Build history of the part. All positions in model axes, mm. Face numbers are marked on the shaded views. Round coordinates to 2 decimals unless told otherwise and drop trailing zeros. Loops run counter-clockwise (first coordinate to the right, second up) from the corner with the lowest first, then second, coordinate; pieces in that order, holes last. Notation, with made-up numbers: (50.25, -3) - (74.25, -3) arc R25 cw to (74.25, 21) - close; hole circle Ø6 at (-17, -36.75). An arc over 180 degrees is marked (long way). Use a Markdown table: item, result.
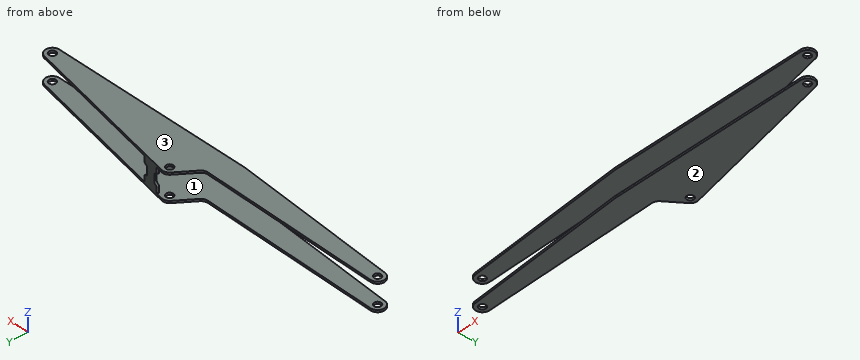
from build123d import *

# Parameters (mm, degrees)
PROFILE_EXTRUDE_DEPTH        = 40
LIGHTNING_BOLT_FILLET_R      = 10
SHELL_CUT_REACH              = 291.378
SHELL_SKETCH_W               = 549.904110801
SHELL_SKETCH_H               = 34
HOLES_START                  = -40
HOLES_SKETCH_R               = 5
HOLES_CUT_DEPTH              = 40
BOWTIE_SUPPORT_EXTRUDE_DEPTH = 3
BOWTIE_SUPPORT_FILLET_R      = 2.5


# Some blends are built 0.0001 mm under size
with BuildPart() as part:
    # Profile Sketch → Profile Extrude (new body)
    with BuildSketch(Plane.XY):
        with BuildLine():
            Line((-25, -34.499500189), (-265.820932486, -14.965628235))
            ThreePointArc((-265.820932486, -14.965628235), (-275, -4.499500189), (-264.823685281, 4.999854285))
            Line((-264.823685281, 4.999854285), (0, 0))
            Line((0, 0), (25, 34.499500189))
            Line((25, 34.499500189), (267.042170119, -14.699900238))
            ThreePointArc((267.042170119, -14.699900238), (275, -25.500499811), (265.050226145, -34.499500189))
            Line((265.050226145, -34.499500189), (-25, -34.499500189))
        make_face()
    extrude(amount=PROFILE_EXTRUDE_DEPTH)

    # Lightning Bolt Fillet
    # the kernel refuses this fillet: 10 mm, written as the material it adds along each edge
    with BuildSketch(Plane(origin=(0, 0, 0), x_dir=(-0.9998218216369521, 0.0188765722144361, 0), z_dir=(0, 0, 1))) as lightning_bolt_fillet_piece_1:
        with BuildLine():
            CenterArc((LIGHTNING_BOLT_FILLET_R * 0.522262066694, -LIGHTNING_BOLT_FILLET_R), LIGHTNING_BOLT_FILLET_R, 90, 55.152715338)
            Line((-LIGHTNING_BOLT_FILLET_R * 0.298415868343, -LIGHTNING_BOLT_FILLET_R * 0.428608954443), (0, 0))
            Line((0, 0), (LIGHTNING_BOLT_FILLET_R * 0.522262066694, 0))
        make_face()
    extrude(amount=40)
    # the kernel refuses this fillet: 10 mm, written as the material it takes off along each edge
    with BuildSketch(Plane(origin=(25, 34.499500189, -16.099347603), x_dir=(0.9799599951405409, -0.19919439732118757, 0), z_dir=(0, 0, 1))) as lightning_bolt_fillet_2_piece_1:
        with BuildLine():
            CenterArc((LIGHTNING_BOLT_FILLET_R * 0.643973904117, -LIGHTNING_BOLT_FILLET_R), LIGHTNING_BOLT_FILLET_R, 90, 65.560956721)
            Line((-LIGHTNING_BOLT_FILLET_R * 0.266428041961, -LIGHTNING_BOLT_FILLET_R * 0.586275095532), (0, 0))
            Line((0, 0), (LIGHTNING_BOLT_FILLET_R * 0.643973904117, 0))
        make_face()
    extrude(amount=72.198695206, mode=Mode.SUBTRACT)
    with BuildSketch(Plane(origin=(-25, -34.499500189, -1.012258703), x_dir=(1, 0, 0), z_dir=(0, 0, 1))) as lightning_bolt_fillet_2_piece_2:
        with BuildLine():
            CenterArc((LIGHTNING_BOLT_FILLET_R * 0.0404903481386, LIGHTNING_BOLT_FILLET_R), LIGHTNING_BOLT_FILLET_R, 265.36268102, 4.63731898)
            Line((-LIGHTNING_BOLT_FILLET_R * 0.040357800163, LIGHTNING_BOLT_FILLET_R * 0.0032735696711), (0, 0))
            Line((0, 0), (LIGHTNING_BOLT_FILLET_R * 0.0404903481386, 0))
        make_face()
    extrude(amount=42.024517407, mode=Mode.SUBTRACT)

    # Shell Cut: up to this plane
    shell_cut_end = Plane(origin=(25, 34.499500189, 40), z_dir=(-0.19919439732118804, -0.9799599951405409, 0))
    # Shell Sketch → Shell Cut (cut, up to the surface)
    with BuildSketch(Plane(origin=(-2.943500576, -36.288584016, 0), x_dir=(0.996726430328903, -0.080848148301631, 0), z_dir=(-0.080848148301631, -0.996726430328903, 0)), mode=Mode.PRIVATE) as shell_cut_sk1:
        with Locations((1.211249587, 20)):
            Rectangle(SHELL_SKETCH_W, SHELL_SKETCH_H)
    shell_cut_tool1 = split(extrude(shell_cut_sk1.sketch, amount=-SHELL_CUT_REACH, mode=Mode.PRIVATE), bisect_by=shell_cut_end, keep=Keep.BOTH, mode=Mode.PRIVATE)
    add(shell_cut_tool1.solids().sort_by_distance((-1.736216, -36.386511, 20))[0], mode=Mode.SUBTRACT)


with BuildPart() as shell_cut_piece_1:
    # of the separate pieces the step leaves, piece 1, a body of its own (shell_cut_pieces)
    add(part.part.solids().sort_by_distance((3.06453365, 4.228995169, 37))[0])


with BuildPart() as shell_cut_piece_2:
    # of the separate pieces the step leaves, piece 2, a body of its own (shell_cut_pieces)
    add(part.part.solids().sort_by_distance((-5.221690109, 0.098585176, 0))[0])


with BuildPart() as holes_cut_tool:
    # Holes Sketch → Holes Cut (new body)
    with BuildSketch(Plane.XY.offset(40).offset(HOLES_START)):
        with Locations((-265.012451003, -4.998363931)):
            Circle(HOLES_SKETCH_R)
        with Locations((29.318742666, 23.4171403)):
            Circle(HOLES_SKETCH_R)
        with Locations((265.050226145, -24.499500189)):
            Circle(HOLES_SKETCH_R)
    extrude(amount=HOLES_CUT_DEPTH)


with BuildPart() as shell_cut_piece_1_1:
    add(shell_cut_piece_1.part)

    # Holes Cut: cut by holes_cut_tool
    add(holes_cut_tool.part, mode=Mode.SUBTRACT)



with BuildPart() as shell_cut_piece_2_1:
    add(shell_cut_piece_2.part)

    # Holes Cut: cut by holes_cut_tool
    add(holes_cut_tool.part, mode=Mode.SUBTRACT)


with BuildPart() as shell_cut_piece_1_2:
    add(shell_cut_piece_1_1.part)

    add(shell_cut_piece_2_1.part)  # Bowtie Support Extrude merges Shell Cut piece 2
    # Bowtie Support Sketch → Bowtie Support Extrude (add)
    with BuildSketch(Plane(origin=(7.726350286, 38.010678463, 0), x_dir=(0.9799599951405408, -0.1991943973211881, 0), z_dir=(0.1991943973211881, 0.9799599951405409, 0))):
        Polygon((39.066631772, -27), (39.066631772, -13), (34.066631772, -13), (34.066631772, -3), (39.066631772, -3), (54.066631772, -3), (59.066631772, -3), (59.066631772, -13), (54.066631772, -13), (54.066631772, -27), (59.066631772, -27), (59.066631772, -37), (54.066631772, -37), (39.066631772, -37), (34.066631772, -37), (34.066631772, -27), align=None)
    extrude(amount=-BOWTIE_SUPPORT_EXTRUDE_DEPTH)

    # Bowtie Support Fillet
    bowtie_support_fillet_edges = [shell_cut_piece_1_2.edges().sort_by_distance(p)[0] for p in [
        (60.410694898, 25.77096834, 13),
        (60.410694898, 25.77096834, 27),
        (45.711294971, 28.758884299, 13),
        (45.711294971, 28.758884299, 27),
    ]]
    fillet(bowtie_support_fillet_edges, radius=BOWTIE_SUPPORT_FILLET_R)
    bowtie_support_fillet_2_edges = [shell_cut_piece_1_2.edges().sort_by_distance(p)[0] for p in [
        (65.310494873, 24.774996353, 13),
        (65.310494873, 24.774996353, 27),
        (40.811494995, 29.754856286, 13),
        (40.811494995, 29.754856286, 27),
    ]]
    fillet(bowtie_support_fillet_2_edges, radius=BOWTIE_SUPPORT_FILLET_R - 0.0001)  # a hair under: the kernel refuses the full size


solid = shell_cut_piece_1_2.part
Q1. Pull direction Z, two halves, no side cores. Call the marked faces 1, 2 and 3: pulls with the +Z half, pulls with the -Z half, needs draft (parallel to the pull), parting line crosses it, or undercut.
Results found:
| item | result |
|---|---|
| face 1 | undercut |
| face 2 | pulls with the -Z half |
| face 3 | pulls with the +Z half |
Q2. Cut at B-B, the plane x = 190.5. List the corners of the cut face in (y, z).
Results found:
| item | result |
|---|---|
| outline | (-34.5, 0) - (0.86, 0) - (0.86, 3) - (-34.5, 3) - close; (-34.5, 37) - (0.86, 37) - (0.86, 40) - (-34.5, 40) - close |
Q3. Drop flat-ended pins along their axis: pin 1 (9 mm diameter, centred on x = -265.01, y = -5, fed in from -Z); pin 2 (0.5 mm diameter, centred on x = 43.5, y = 30, fed in from -Z). Give the stop position or say it passes through.
Results found:
| item | result |
|---|---|
| pin 1 | passes through |
| pin 2 | stops at z = 0 |
Q4. Probe line 1 (Z direction, x = -2.5, y = -7.5); line 2 (Y direction, x = 220, z = 38); line 3 (Y direction, x = 79, z = 38). List the from-to ranges inside material, lowest first.
Results found:
| item | result |
|---|---|
| line 1 | z = 0 to 3, 37 to 40 |
| line 2 | y = -34.5 to -5.14 |
| line 3 | y = -34.5 to 23.52 |
Q5. Cut at A-A, the plane x = -54.5. List the corners of the cut face in (y, z), plus the area to 3 significant figures.
Results found:
| item | result |
|---|---|
| outline | (-32.11, 0) - (1.03, 0) - (1.03, 3) - (-32.11, 3) - close; (-32.11, 37) - (1.03, 37) - (1.03, 40) - (-32.11, 40) - close |
| area | 199 mm2 |
